Geometry check sheet. Reference: the model listing, model coordinates, mm. A direction names the side the tool comes from. Round coordinates to 2 decimals unless told otherwise and drop trailing zeros. Order: outer loops, then holes, each group sorted by start corner. A loop starts at its lowest first (then second) coordinate and runs counter-clockwise, first axis right, second up. Notation, with made-up numbers: (70.25, -15.5) -> (128.25, -15.5) arc R25 ccw to (128.25, 3.5) -> close; hole circle Ø11 at (5, 69). An arc over 180 degrees is marked (long way). Use a Markdown table: item, result. Add a question column.
Item 1: Mould release check, pull along Y, two halves, no side actions. Record for faces 1 (the flat face through (-1, -21.875, 34)), 2 (the cylindrical face through (73.147, 18.208, 33.726)): pulls with the +Y half, pulls with the -Y half, needs draft (parallel to the pull), parting line crosses it, or undercut.
Item 2: Sectioned sample at B-B, the plane z = 33.65. State how many separate pieces and enclosed holes the cut face has, and give its area (3 significant figures).
Item 3: Sectioned sample at A-A, the plane x = 71.25. Record the cut outline in (y, z) (3 decimals), and give its area (3 significant figures).
Item 4: Material ranges on probe 1 along X at (y, z) = (-6, 34); probe 2 along Y at (x, z) = (18, 32.7) (3 decimals); probe 3 along Y at (x, z) = (23.75, 33.1) (3 decimals), recorded low to high. Write a range as [from, to].
Item 5: Set-up check for faces 3 (the flat face through (-56, 1.125, 34)), 4 (the cylindrical face through (93.496, -20.449, 33.774)): record each of +Z, -Z, +X, -X, +Y, -Y from which the full face is reachable in a straight line by a thin tool's end or side.
from build123d import *

# Parameters (mm, degrees)
SKETCH1_W             = 190
SKETCH1_H             = 43.75
BOSS_EXTRUDE1_DEPTH   = 3.5
F_6_CLEARANCE_HOLE1_D = 3.7973
CUT_EXTRUDE1_DEPTH    = 98.548785871
FILLET1_R             = 2
FILLET2_R             = 5
F_6_CLEARANCE_HOLE2_D = 3.556


with BuildPart() as part:
    # Sketch1 → Boss-Extrude1 (new body)
    with BuildSketch(Plane.XY.offset(32)):
        Rectangle(SKETCH1_W, SKETCH1_H)
    extrude(amount=BOSS_EXTRUDE1_DEPTH)

    # #6 Clearance Hole1 (through all)
    with Locations(Plane.XY.offset(35.5)):
        with Locations((71.25, 18.125), (23.75, 18.125), (-23.75, 18.125), (-71.25, 18.125), (-71.25, -18.125), (-23.75, -18.125), (23.75, -18.125), (71.25, -18.125)):
            Hole(F_6_CLEARANCE_HOLE1_D / 2)

    # Sketch6 → Cut-Extrude1 (cut, through all)
    with BuildSketch(Plane.XY.offset(35.5)):
        with BuildLine():
            Line((36.468626967, -7.875), (41.5, -7.875))
            Line((41.5, -7.875), (41.5, 1.125))
            Line((41.5, 1.125), (36.468626967, 1.125))
            ThreePointArc((36.468626967, 1.125), (32.5, 2.625), (28.531373033, 1.125))
            Line((28.531373033, 1.125), (23.5, 1.125))
            Line((23.5, 1.125), (23.5, -7.875))
            Line((23.5, -7.875), (28.531373033, -7.875))
            ThreePointArc((28.531373033, -7.875), (32.5, -9.375), (36.468626967, -7.875))
        make_face()
        with BuildLine():
            Line((-70.5, 1.125), (-70.5, -7.875))
            Line((-70.5, -7.875), (-65.468626967, -7.875))
            ThreePointArc((-65.468626967, -7.875), (-61.5, -9.375), (-57.531373033, -7.875))
            Line((-57.531373033, -7.875), (-52.5, -7.875))
            Line((-52.5, -7.875), (-52.5, 1.125))
            Line((-52.5, 1.125), (-57.531373033, 1.125))
            ThreePointArc((-57.531373033, 1.125), (-61.5, 2.625), (-65.468626967, 1.125))
            Line((-65.468626967, 1.125), (-70.5, 1.125))
        make_face()
    extrude(amount=-CUT_EXTRUDE1_DEPTH, mode=Mode.SUBTRACT)

    # Fillet1
    fillet1_edges = [part.edges().sort_by_distance(p)[0] for p in [
        (41.5, 1.125, 33.75),
        (41.5, -7.875, 33.75),
        (23.5, -7.875, 33.75),
        (23.5, 1.125, 33.75),
        (-52.5, 1.125, 33.75),
        (-52.5, -7.875, 33.75),
        (-70.5, -7.875, 33.75),
        (-70.5, 1.125, 33.75),
    ]]
    fillet(fillet1_edges, radius=FILLET1_R)

    # Fillet2
    fillet2_edges = [part.edges().sort_by_distance(p)[0] for p in [
        (95, -21.875, 33.75),
        (-95, -21.875, 33.75),
        (-95, 21.875, 33.75),
        (95, 21.875, 33.75),
    ]]
    fillet(fillet2_edges, radius=FILLET2_R)

    # #6 Clearance Hole2 (through all)
    with Locations(Plane.XY.offset(35.5)):
        with Locations((78, 0), (48, 0), (18, 0), (-18, 0), (-48, 0), (-78, 0)):
            Hole(F_6_CLEARANCE_HOLE2_D / 2)


solid = part.part
Found:
| question | item | result |
|---|---|---|
| 1 | face 1 | pulls with the -Y half |
| 1 | face 2 | undercut |
| 2 | separate pieces | 1 |
| 2 | enclosed holes | 16 |
| 2 | area | 7,790 mm2 |
| 3 | outline | (-21.875, 32) -> (-20.024, 32) -> (-20.024, 35.5) -> (-21.875, 35.5) -> close; (-16.226, 32) -> (16.226, 32) -> (16.226, 35.5) -> (-16.226, 35.5) -> close; (20.024, 32) -> (21.875, 32) -> (21.875, 35.5) -> (20.024, 35.5) -> close |
| 3 | area | 127 mm2 |
| 4 | probe 1 | x = [-95, -70.5], [-52.5, 23.5], [41.5, 95] |
| 4 | probe 2 | y = [-21.875, -1.778], [1.778, 21.875] |
| 4 | probe 3 | y = [-21.875, -20.024], [-16.226, -6.843], [0.093, 16.226], [20.024, 21.875] |
| 5 | face 3 | +Z, -Z |
| 5 | face 4 | +Z, -Z, +X, -Y |
